Design review of the part built by this model. Coordinates are the model's own, in mm. A direction names the side the tool comes from. Round coordinates to 2 decimals unless told otherwise and drop trailing zeros. Return JSON: item names as keys, results as strings. Group by question number.
(1) For faces 1 (the cylindrical face through (2.53, -57.08, 79.98)), 2 (the cylindrical face through (9.821, -57.325, 68.767)), list the 3-axis set-ups (+Z, -Z, +X, -X, +Y, -Y) from which the entire face can be reached by the end or side of a thin tool; tool diameter is ignored.
(2) Clearance check with flat-ended pins moving along their axes: pin 1 (2 mm diameter, centred on x = -2.5, z = 54.5, fed in from +Y); pin 2 (2 mm diameter, centred on x = 1.5, y = -48, fed in from +Z); pin 3 (1 mm diameter, centred on x = -3, y = -47, fed in from -Z); pin 4 (2.5 mm diameter, centred on y = -115.56, z = 47.52, fed in from -X). State where each tip first meets the part, or that it passes through.
(3) The part is to be moulded in two halves that separate along X. For faces 3 (the flat face through (7.095, -58, 70)), 4 (the flat face through (-7.405, -52, 70)), 5 (the flat face through (-1.905, -59, 70)), 6 (the cylindrical face through (-4.679, -57.325, 68.767)), say which applies: pulls with the +X half, pulls with the -X half, needs draft (parallel to the pull), parting line crosses it, or undercut.
(4) Wall thickness on L1, parallel to Y at x = 5, z = 68; L2, parallel to X at y = 11.5, z = 19.5; L3, parallel to Y at x = 7.5, z = 60.5: over which ranges is each line inside the solid? List them lowest first. Write a range as [from, to].
from build123d import *

# Parameters (mm, degrees)
REVOLVE1_ANGLE          = 180
BOSS_EXTRUDE5_START     = -20
BOSS_EXTRUDE5_OUTLINE_R = 1.45
BOSS_EXTRUDE5_DEPTH     = 20
FILLET1_R               = 1
FILLET2_R               = 1
FILLET3_R               = 1


# Read off the part's stored shape, not the designer's step: Boss-Extrude5
with BuildPart() as part:
    # Sketch1 → Revolve1 (revolve)
    with BuildSketch(Plane.XY):
        with BuildLine():
            Line((-7.404589955, 9.946191987), (-7.404589955, 29.946191987))
            Line((-7.404589955, 29.946191987), (1.095410045, 29.946191987))
            ThreePointArc((1.095410045, 29.946191987), (2.595410045, 28.446191987), (4.095410045, 29.946191987))
            Line((4.095410045, 29.946191987), (12.595410045, 29.946191987))
            Line((12.595410045, 29.946191987), (12.595410045, 9.946191987))
            Line((12.595410045, 9.946191987), (7.095410045, 9.946191987))
            Line((7.095410045, 9.946191987), (7.095410045, 21.162110611))
            Line((7.095410045, 21.162110611), (-1.904589955, 21.162110611))
            Line((-1.904589955, 21.162110611), (-1.904589955, 9.946191987))
            Line((-1.904589955, 9.946191987), (-7.404589955, 9.946191987))
        make_face()
    revolve(axis=Axis((-85.384931054, -58.837889389, 0), (1, 0, 0)), revolution_arc=REVOLVE1_ANGLE)

    # Boss-Extrude5 outline → Boss-Extrude5 (cut)
    with BuildSketch(Plane.ZY.offset(7.404589955).offset(BOSS_EXTRUDE5_START)):
        with Locations((25.365468004, 10.67896492)):
            Circle(BOSS_EXTRUDE5_OUTLINE_R)
        with Locations((47.520651548, -115.563436336)):
            Circle(BOSS_EXTRUDE5_OUTLINE_R)
        with Locations((72.886064731, -46.046424732)):
            Circle(BOSS_EXTRUDE5_OUTLINE_R)
        with Locations((56.725485337, -11.317164297)):
            Circle(BOSS_EXTRUDE5_OUTLINE_R)
        with Locations((69.516903931, -84.203221399)):
            Circle(BOSS_EXTRUDE5_OUTLINE_R)
        with Locations((12.791101566, -131.723684009)):
            Circle(BOSS_EXTRUDE5_OUTLINE_R)
    extrude(amount=BOSS_EXTRUDE5_DEPTH, mode=Mode.SUBTRACT)

    # Fillet1
    fillet1_edges = [part.edges().sort_by_distance(p)[0] for p in [
        (12.595410045, -58.837889389, 88.784081376),
    ]]
    fillet(fillet1_edges, radius=FILLET1_R)

    # Fillet2
    fillet2_edges = [part.edges().sort_by_distance(p)[0] for p in [
        (-7.404589955, -58.837889389, 88.784081376),
    ]]
    fillet(fillet2_edges, radius=FILLET2_R)

    # Fillet3
    fillet3_edges = [part.edges().sort_by_distance(p)[0] for p in [
        (-7.404589955, -58.837889389, 68.784081376),
        (12.595410045, -58.837889389, 68.784081376),
        (7.095410045, -58.837889389, 68.784081376),
        (-1.904589955, -58.837889389, 68.784081376),
    ]]
    fillet(fillet3_edges, radius=FILLET3_R)


solid = part.part
Solutions:
{
 "1": {"face 1": "-Z", "face 2": "-Z, +X, -X"},
 "2": {"pin 1": "y = 12.02", "pin 2": "z = 88.23", "pin 3": "z = 67.67", "pin 4": "through"},
 "3": {"face 3": "undercut", "face 4": "pulls with the -X half", "face 5": "undercut", "face 6": "needs draft"},
 "4": {"L1": "[-115.92, -100.98], [-16.7, -1.75]", "L2": "[-7.4, -1.9], [7.1, 12.6]", "L3": "[-123.82, -91.98], [-25.7, 6.14]"}
}
